from build123d import *

# Parameters (mm, degrees)
BOSS_EXTRU_1_DEPTH                                = 1.5
ESQUISSE2_W                                       = 4
ESQUISSE2_H                                       = 2.5
CHAMBRAGE_POUR_VIS_T_TE_HEXAGONALE_M2_D           = 3
CHAMBRAGE_POUR_VIS_T_TE_HEXAGONALE_M2_DEPTH       = 4
CHAMBRAGE_POUR_VIS_T_TE_HEXAGONALE_M2_CBORE_D     = 5
CHAMBRAGE_POUR_VIS_T_TE_HEXAGONALE_M2_CBORE_DEPTH = 2.5
CHANFREIN1_SIZE                                   = 0.66150504
CHANFREIN1_SIZE2                                  = 0.116617787


with BuildPart() as part:
    # Esquisse1 → Boss.-Extru.1 (new body)
    with BuildSketch(Plane.XY):
        Polygon((-27.097787955, 20.402380339), (-22.922211673, 17.509970722), (-23.817460632, 22.509970718), (-18.739232742, 22.624304328), (-22.402430623, 26.143175168), (-18.36126158, 29.220580467), (-23.393191293, 29.914233086), (-21.932670307, 34.779245838), (-26.411305743, 32.382728509), (-28.089302186, 37.177079198), (-30.303956824, 32.605780103), (-34.479533107, 35.49818972), (-33.584284152, 30.498189734), (-38.662512037, 30.383856115), (-34.999314157, 26.864985274), (-39.040483199, 23.787579976), (-34.008553486, 23.093927357), (-35.469074473, 18.228914604), (-30.990439036, 20.625431934), (-29.312442593, 15.831081245), align=None)
    extrude(amount=-BOSS_EXTRU_1_DEPTH)

    # Esquisse2 → Révolution1 (revolve)
    with BuildSketch(Plane.XZ.offset(-26.504080221)):
        with Locations((-26.70087239, 1.25)):
            Rectangle(ESQUISSE2_W, ESQUISSE2_H)
    revolve(axis=Axis((-28.70087239, 26.504080221, 2.5), (0, 0, -1)))

    # Chambrage pour vis à tête hexagonale M2.51
    with Locations(Plane.XY.offset(2.5)):
        with Locations((-28.70087239, 26.504080221)):
            CounterBoreHole(CHAMBRAGE_POUR_VIS_T_TE_HEXAGONALE_M2_D / 2, CHAMBRAGE_POUR_VIS_T_TE_HEXAGONALE_M2_CBORE_D / 2, CHAMBRAGE_POUR_VIS_T_TE_HEXAGONALE_M2_CBORE_DEPTH, depth=CHAMBRAGE_POUR_VIS_T_TE_HEXAGONALE_M2_DEPTH)

    # Chanfrein1
    chanfrein1_edges = [part.edges().sort_by_distance(p)[0] for p in [
        (-23.817460632, 22.509970718, -0.75),
    ]]
    chanfrein1_side = [part.faces().sort_by_distance(p)[0] for p in [
        (-23.369836152, 20.00997072, -0.75),
    ]]
    chamfer(chanfrein1_edges, length=CHANFREIN1_SIZE, length2=CHANFREIN1_SIZE2, reference=chanfrein1_side[0])


solid = part.part
Design review of the part built by this model. Coordinates are the model's own, in mm. A direction names the side the tool comes from. Round coordinates to 2 decimals unless told otherwise and drop trailing zeros. Loops run counter-clockwise (first coordinate to the right, second up) from the corner with the lowest first, then second, coordinate; pieces in that order, holes last. Notation, with made-up numbers: (20.25, 61) - (51.25, 61) arc R18 cw to (51.25, 70) - close; hole circle Ø10 at (76, 30). An arc over 180 degrees is marked (long way). One line per item, written item: value. Start each with the question number.
1) Draft analysis for pull direction X (two halves, no side actions). For faces 1 (the flat face through (-24.14, 33.6, -0.74)), 2 (the cylindrical face through (-26.855, 30.053, 1.268)), 3 (the flat face through (-36.86, 28.65, -0.74)), 4 (the flat face through (-23.306, 19.654, -0.74)), state which applies: +X half, -X half, draft (parallel to the pull), parting line (faces both ways), or undercut.
2) Consider section D-D on y = 31. Give the boundary of the cut face in (x, z), then the cut area to 3 significant figures.
3) Consider section C-C on x = -32.25. Give the boundary of the cut face in (y, z).
4) To check wall thickness, follow L1, parallel to X at y = 20, z = -0.55; L2, parallel to Z at x = -25.5, y = 19.5; L3, parallel to X at y = 28.5, z = 1.4. State the ranges of each line that lie inside material, in increasing order. Write a range as from..to.
5) Consider section B-B on z = -1.1. Give the boundary of the cut face in (x, y), then the cut area to 3 significant figures.
6) Consider section A-A on y = 25.25. Give the boundary of the cut face in (x, z).
7) For faces 5 (the flat face through (-32.36, 34.03, -0.74)), 6 (the flat face through (-34.729, 20.695, -0.74)), 7 (the flat face through (-28, 25, 0)), 8 (the flat face through (-20.545, 24.359, -0.74)), 9 (the flat face through (-25.039, 18.976, -0.74)), list the 3-axis set-ups (+Z, -Z, +X, -X, +Y, -Y) from which the entire face can be reached by the end or side of a thin tool; tool diameter is ignored.
8) Insertion check: pin 1 Ø3 at (x, y) = (-35.5, 33.5) entering from +Z; pin 2 Ø1.5 at (y, z) = (19.5, 0.5) entering from +X. Each pin has a flat end and moves straight along its axis. Give the tip position at first contact, or say it passes through.
Reported:
1. face 1: undercut
1. face 2: parting line
1. face 3: -X half
1. face 4: +X half
2. outline: (-33.67, -1.5) - (-23.07, -1.5) - (-23.07, 0) - (-33.67, 0) - close
2. area: 15.9 mm^2
3. outline: (19.95, -1.5) - (33.95, -1.5) - (33.95, 0) - (28.35, 0) - (28.35, 2.5) - (24.66, 2.5) - (24.66, 0) - (19.95, 0) - close
4. L1: x = -34.94..-32.16, -30.77..-27.29, -26.52..-23.37
4. L2: z = -1.5..0
4. L3: x = -32.17..-30.21, -27.2..-25.23
5. outline: (-39.04, 23.79) - (-34.01, 23.09) - (-35.47, 18.23) - (-30.99, 20.63) - (-29.31, 15.83) - (-27.1, 20.4) - (-22.92, 17.51) - (-23.7, 21.86) - (-23.7, 22.51) - (-18.74, 22.62) - (-22.4, 26.14) - (-18.36, 29.22) - (-23.39, 29.91) - (-21.93, 34.78) - (-26.41, 32.38) - (-28.09, 37.18) - (-30.3, 32.61) - (-34.48, 35.5) - (-33.58, 30.5) - (-38.66, 30.38) - (-35, 26.86) - close; hole circle Ø3 at (-28.7, 26.5)
5. area: 201 mm^2
6. outline: (-37.12, -1.5) - (-29.52, -1.5) - (-29.52, 0) - (-30.86, 0) - (-30.86, 2.5) - (-32.5, 2.5) - (-32.5, 0) - (-37.12, 0) - close; (-27.88, -1.5) - (-21.47, -1.5) - (-21.47, 0) - (-24.9, 0) - (-24.9, 2.5) - (-26.54, 2.5) - (-26.54, 0) - (-27.88, 0) - close
7. face 5: +Z, -Z, +Y
7. face 6: +Z, -Z, -X
7. face 7: +Z
7. face 8: +Z, -Z, +X
7. face 9: +Z, -Z, -Y
8. pin 1: stops at z = 0
8. pin 2: stops at x = -23.18
